Read the model definition and answer for the solid it produces. Units are mm, in the model's axes. A direction names the side the tool comes from. Coordinates: 2 decimals unless noted, no trailing zeros. Order: outer loops, then holes, each group sorted by start corner. A loop starts at its lowest first (then second) coordinate and runs counter-clockwise, first axis right, second up. Notation, with made-up numbers: (49.5, 36.25) - (55.5, 36.25) arc R17 cw to (55.5, 43.25) - close; hole circle Ø7 at (-2.75, 71). An arc over 180 degrees is marked (long way). Use one line per item in the form item = value. Start each with the question number.
from build123d import *

# Parameters (mm, degrees)
F0_R     = 3
F1_DEPTH = 1.5
F2_SIZE  = 1.49999
F3_DEPTH = 19.3


# Not quite as in the source:
# - a fillet or chamfer is up to 0.001 mm smaller than in the source, because OpenCascade refuses the exact size


with BuildPart() as f1:
    # F0 (on Top) → F1 (new body)
    with BuildSketch(Plane.XY):
        Circle(F0_R)
    extrude(amount=F1_DEPTH)

    # F2 (size 1.5 in the source; OpenCascade refuses exactly that, so slightly less here)
    f2_edges = [f1.edges().sort_by_distance(p)[0] for p in [
        (-3, 0, 1.5),
    ]]
    chamfer(f2_edges, length=F2_SIZE)

    # F3 (add): a face of the model
    f3_faces = [f1.faces().sort_by_distance(p)[0] for p in [
        (0, 0, 1.5),
    ]]
    extrude(f3_faces, amount=F3_DEPTH)


solid = f1.part
Q1. Which of the six approach directions +Z, -Z, +X, -X, +Y, -Y give full straight-line access (tool end or side, diameter ignored) to faces 1 (the flat face through (0, 0, 20.8)), 2 (the cylindrical face through (-0.195, 1.487, 11.015))?
Q2. Consider probe 1 along Y at (x, z) = (-0.9, 16.5); probe 2 along X at (y, z) = (1.25, 4). Determine where each line is inside the solid, lowest interval first.
Q3. Given P1, Ø2, axis at x = 1.5, z = 18, coming from the +Y side, flat-ended and moving along its own axis, determine where the tip first touches the part or whether it passes through.
Q4. A cutting plane is placed at C-C (z = 8.5). Give the vertices of the cut face in (x, y), then the cut area to 3 significant figures.
Result sheet:
q1.face_1 = +Z, +X, -X, +Y, -Y
q1.face_2 = +Z
q2.probe_1 = -1.2 to 1.2
q2.probe_2 = -0.83 to 0.83
q3.P1 = 1.41
q4.outline = circle Ø3 at (0, 0)
q4.area = 7.07 mm^2
